Here's how the part is built. I have some questions about the finished solid (model axes, mm). Coordinates: 2 decimals unless noted, no trailing zeros. Write each loop counter-clockwise with the first axis right and the second up, starting at its lowest first coordinate (ties: lowest second). Pieces come first, ordered by that corner, then holes.
Item 1: If we section it at B-B (x = 59): Please give me the cut outline in (y, z), then the cut area to 3 significant figures.
Item 2: If we section it at C-C (y = 85): Please give me the cut outline in (x, z), then the cut area to 3 significant figures.
Item 3: If I drill on line 1 (Y direction, x = 104.5, z = 3.15); line 2 (Y direction, x = 10, z = 1.35) (3 decimals); line 3 (Y direction, x = -23, z = 2), over which ranges is the centre line in solid material (lowest first)?
Item 4: I'm going to push flat-ended pins straight in: pin 1 Ø8 at (x, y) = (86.5, 64) entering from -Z; pin 2 Ø1.2 at (x, z) = (-49.5, 1.5) entering from +Y; pin 3 Ø2 at (x, z) = (50.5, 2.5) entering from -Y. Where does each tip first touch, or does it pass through?
Item 5: If we section it at D-D (z = -12.25): Please give me the cut outline in (x, y).
Item 6: If we section it at A-A (y = 46.5): Please give me the cut outline in (x, z).
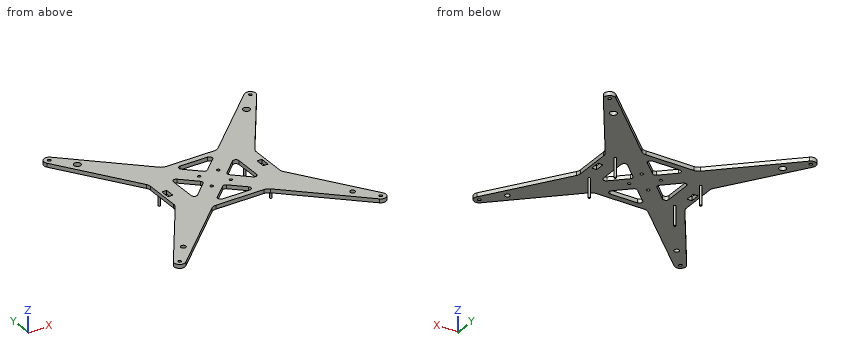
from build123d import *

# Parameters (mm, degrees)
F0_R     = 1.65
F0_R_2   = 2.55
F0_R_3   = 1.525
F0_W     = 5
F0_H     = 10
F0_R_4   = 3.555
F1_DEPTH = 4
F2_R     = 1
F3_DEPTH = 20
F4_R     = 3.555
F4_R_2   = 2.55
F5_DEPTH = 4


with BuildPart() as f1:
    # F0 (on Top) → F1 (new body)
    with BuildSketch(Plane.XY):
        with BuildLine():
            ThreePointArc((-56.363239, 23.1312), (-55.348378, 20.999418), (-54.999976, 18.664241))
            Line((-54.999976, 18.664241), (-54.999976, -18.664242))
            ThreePointArc((-54.999976, -18.664242), (-55.348378, -20.999419), (-56.363239, -23.1312))
            Line((-56.363239, -23.1312), (-109.062757, -101.428966))
            ThreePointArc((-109.062757, -101.428966), (-108.056825, -108.695115), (-100.723998, -108.498976))
            Line((-100.723998, -108.498976), (-30.492366, -42.183308))
            ThreePointArc((-30.492366, -42.183308), (-27.955204, -40.565838), (-25, -40))
            Line((-25, -40), (25, -40))
            ThreePointArc((25, -40), (27.955204, -40.565838), (30.492367, -42.183308))
            Line((30.492367, -42.183308), (100.723998, -108.498976))
            ThreePointArc((100.723998, -108.498976), (108.056825, -108.695115), (109.062757, -101.428966))
            Line((109.062757, -101.428966), (56.363239, -23.1312))
            ThreePointArc((56.363239, -23.1312), (55.348379, -20.999418), (54.999977, -18.664242))
            Line((54.999977, -18.664242), (54.999977, 18.664241))
            ThreePointArc((54.999977, 18.664241), (55.348379, 20.999418), (56.363239, 23.1312))
            Line((56.363239, 23.1312), (109.062757, 101.428966))
            ThreePointArc((109.062757, 101.428966), (108.056825, 108.695115), (100.723998, 108.498976))
            Line((100.723998, 108.498976), (30.492367, 42.183307))
            ThreePointArc((30.492367, 42.183307), (27.955204, 40.565837), (25, 40))
            Line((25, 40), (-25, 40))
            ThreePointArc((-25, 40), (-27.955204, 40.565837), (-30.492366, 42.183307))
            Line((-30.492366, 42.183307), (-100.723998, 108.498976))
            ThreePointArc((-100.723998, 108.498976), (-108.056825, 108.695115), (-109.062757, 101.428966))
            Line((-109.062757, 101.428966), (-56.363239, 23.1312))
        make_face()
        with Locations((-104.5, -104.5)):
            Circle(F0_R, mode=Mode.SUBTRACT)
        with Locations((-87.96694, -85)):
            Circle(F0_R_2, mode=Mode.SUBTRACT)
        with Locations((-44.444976, -20.807752)):
            Circle(F0_R_2, mode=Mode.SUBTRACT)
        with BuildLine():
            ThreePointArc((-34, 14.278979), (-32.187663, 17.033876), (-28.940362, 16.460239))
            Line((-28.940362, 16.460239), (-13.818204, 2.181259))
            ThreePointArc((-13.818204, 2.181259), (-12.877841, -1e-06), (-13.818204, -2.18126))
            Line((-13.818204, -2.18126), (-28.940362, -16.460239))
            ThreePointArc((-28.940362, -16.460239), (-32.187663, -17.033877), (-34, -14.27898))
            Line((-34, -14.27898), (-34, 14.278979))
        make_face(mode=Mode.SUBTRACT)
        with Locations((-10, -10)):
            Circle(F0_R_3, mode=Mode.SUBTRACT)
        with Locations((104.5, -104.5)):
            Circle(F0_R, mode=Mode.SUBTRACT)
        with Locations((87.966941, -85)):
            Circle(F0_R_2, mode=Mode.SUBTRACT)
        with BuildLine():
            ThreePointArc((-14.278979, -34), (-17.06679, -32.108202), (-16.338617, -28.818741))
            Line((-16.338617, -28.818741), (-2.059637, -15.335926))
            ThreePointArc((-2.059637, -15.335926), (0, -14.517186), (2.059638, -15.335926))
            Line((2.059638, -15.335926), (16.338617, -28.818741))
            ThreePointArc((16.338617, -28.818741), (17.06679, -32.108202), (14.27898, -34))
            Line((14.27898, -34), (-14.278979, -34))
        make_face(mode=Mode.SUBTRACT)
        with Locations((10, -10)):
            Circle(F0_R_3, mode=Mode.SUBTRACT)
        with Locations((44.444977, -20.807752)):
            Circle(F0_R_2, mode=Mode.SUBTRACT)
        with Locations((-49.499976, 0)):
            Rectangle(F0_W, F0_H, mode=Mode.SUBTRACT)
        with Locations((-44.444976, 20.810818)):
            Circle(F0_R_4, mode=Mode.SUBTRACT)
        with Locations((-10, 10)):
            Circle(F0_R_3, mode=Mode.SUBTRACT)
        with Locations((-87.96694, 85)):
            Circle(F0_R_4, mode=Mode.SUBTRACT)
        with Locations((-104.5, 104.5)):
            Circle(F0_R, mode=Mode.SUBTRACT)
        with Locations((10, 10)):
            Circle(F0_R_3, mode=Mode.SUBTRACT)
        with BuildLine():
            ThreePointArc((28.940363, 16.460239), (32.187664, 17.033876), (34, 14.278979))
            Line((34, 14.278979), (34, -14.27898))
            ThreePointArc((34, -14.27898), (32.187663, -17.033876), (28.940363, -16.460239))
            Line((28.940363, -16.460239), (13.818205, -2.18126))
            ThreePointArc((13.818205, -2.18126), (12.877842, 0), (13.818205, 2.181259))
            Line((13.818205, 2.181259), (28.940363, 16.460239))
        make_face(mode=Mode.SUBTRACT)
        with BuildLine():
            ThreePointArc((14.27898, 34), (17.066791, 32.108201), (16.338617, 28.81874))
            Line((16.338617, 28.81874), (2.059638, 15.335925))
            ThreePointArc((2.059638, 15.335925), (0, 14.517185), (-2.059637, 15.335925))
            Line((-2.059637, 15.335925), (-16.338617, 28.81874))
            ThreePointArc((-16.338617, 28.81874), (-17.06679, 32.108201), (-14.278979, 34))
            Line((-14.278979, 34), (14.27898, 34))
        make_face(mode=Mode.SUBTRACT)
        with Locations((49.499977, 0)):
            Rectangle(F0_W, F0_H, mode=Mode.SUBTRACT)
        with Locations((44.444977, 20.810818)):
            Circle(F0_R_4, mode=Mode.SUBTRACT)
        with Locations((87.966941, 85)):
            Circle(F0_R_4, mode=Mode.SUBTRACT)
        with Locations((104.5, 104.5)):
            Circle(F0_R, mode=Mode.SUBTRACT)
    extrude(amount=F1_DEPTH)



with BuildPart() as f3:
    # F2 (on Top) → F3 (new body)
    with BuildSketch(Plane.XY):
        with Locations((-44.444976, 20.810818)):
            Circle(F2_R)
        with Locations((-44.444976, -20.807752)):
            Circle(F2_R)
        with Locations((44.444977, 20.810818)):
            Circle(F2_R)
        with Locations((44.444977, -20.807752)):
            Circle(F2_R)
    extrude(amount=-F3_DEPTH)


with BuildPart() as f1_1:
    add(f1.part)

    add(f3.part)  # F5 merges F3
    # F4 (on face) → F5 (join)
    with BuildSketch(Plane.XY.offset(4)):
        with Locations((44.444977, 20.810818)):
            Circle(F4_R)
        with Locations((44.444977, -20.807752)):
            Circle(F4_R_2)
        with Locations((-44.444976, -20.807752)):
            Circle(F4_R_2)
        with Locations((-44.444976, 20.810818)):
            Circle(F4_R)
    extrude(amount=-F5_DEPTH)


solid = f1_1.part
Answer list:
1. outline: (-69.1, 0) - (-27.05, 0) - (-27.05, 4) - (-69.1, 4) - close; (27.05, 0) - (69.1, 0) - (69.1, 4) - (27.05, 4) - close
1. area: 336 mm2
2. outline: (-98, 0) - (-91.52, 0) - (-91.52, 4) - (-98, 4) - close; (-84.41, 0) - (-75.84, 0) - (-75.84, 4) - (-84.41, 4) - close; (75.84, 0) - (84.41, 0) - (84.41, 4) - (75.84, 4) - close; (91.52, 0) - (98, 0) - (98, 4) - (91.52, 4) - close
2. area: 120 mm2
3. line 1: y = -110 to -106.15, -102.85 to -94.65, 94.65 to 102.85, 106.15 to 110
3. line 2: y = -40 to -34, -22.834 to -11.525, -8.475 to 8.475, 11.525 to 22.834, 34 to 40
3. line 3: y = -40 to -10.85, 10.85 to 40
4. pin 1: stops at z = 0
4. pin 2: stops at y = 60.7
4. pin 3: stops at y = -62.02
5. outline: circle Ø2 at (-44.44, -20.81); circle Ø2 at (-44.44, 20.81); circle Ø2 at (44.44, -20.81); circle Ø2 at (44.44, 20.81)
6. outline: (-72.09, 0) - (-35.06, 0) - (-35.06, 4) - (-72.09, 4) - close; (35.06, 0) - (72.09, 0) - (72.09, 4) - (35.06, 4) - close
